```python
from build123d import *

# Parameters (mm, degrees)
BOSS_EXTRUDE1_DEPTH  = 3
SKETCH2_R            = 6
CUT_EXTRUDE1_DEPTH   = 4
M5_CLEARANCE_HOLE1_D = 5.5


with BuildPart() as part:
    # Sketch1 → Boss-Extrude1 (new body)
    with BuildSketch(Plane.XY):
        Polygon((-12.5, 55), (-32.5, 35), (-32.5, 2), (-30.5, 0), (30.5, 0), (32.5, 2), (32.5, 35), (12.5, 55), align=None)
    extrude(amount=BOSS_EXTRUDE1_DEPTH)

    # Sketch2 → Cut-Extrude1 (cut, through all)
    with BuildSketch(Plane.XY):
        with Locations((0, 40)):
            Circle(SKETCH2_R)
    extrude(amount=CUT_EXTRUDE1_DEPTH, mode=Mode.SUBTRACT)

    # M5 Clearance Hole1 (through all)
    with Locations(Plane.XY.offset(3)):
        with Locations((-22.5, 14.5), (22.5, 14.5)):
            Hole(M5_CLEARANCE_HOLE1_D / 2)


solid = part.part
```
Can you work these out from the model? Positions are in its coordinate system, mm. Give positions to 0.01 mm unless a question says otherwise; leave off trailing zeros. Write each loop counter-clockwise with the first axis right and the second up, starting at its lowest first coordinate (ties: lowest second). Pieces come first, ordered by that corner, then holes. Notation, with made-up numbers: (84.5, -13.5) -> (88.5, -13.5) arc R14 cw to (88.5, -4.5) -> close; hole circle Ø1 at (32, 80). An arc over 180 degrees is marked (long way). Write item = value, one per line.
(1) Suppose I cut it at B-B on x = -22.5. Write out the boundary of the cut face in (y, z).
Worked out:
outline = (0, 0) -> (11.75, 0) -> (11.75, 3) -> (0, 3) -> close; (17.25, 0) -> (45, 0) -> (45, 3) -> (17.25, 3) -> close
(2) I'm going to push a flat-ended pin straight in: P1, Ø1.5, axis at x = -20.5, z = 1.5, coming from the +Y side. Where does the tip first touch, or does it pass through?
Worked out:
P1 = 47.75
(3) Suppose I cut it at C-C on z = 1.15. Write out the boundary of the cut face in (x, y), then the cut area to 3 significant figures.
Worked out:
outline = (-32.5, 2) -> (-30.5, 0) -> (30.5, 0) -> (32.5, 2) -> (32.5, 35) -> (12.5, 55) -> (-12.5, 55) -> (-32.5, 35) -> close; hole circle Ø5.5 at (-22.5, 14.5); hole circle Ø12 at (0, 40); hole circle Ø5.5 at (22.5, 14.5)
area = 3,010 mm^2
(4) Suppose I cut it at A-A on y = 40. Write out the boundary of the cut face in (x, z), then the cut area to 3 significant figures.
Worked out:
outline = (-27.5, 0) -> (-6, 0) -> (-6, 3) -> (-27.5, 3) -> close; (6, 0) -> (27.5, 0) -> (27.5, 3) -> (6, 3) -> close
area = 129 mm^2
(5) I need wall thicknesses on probe 1 along X at (y, z) = (12, 1.4); probe 2 along Y at (x, z) = (0, 2.05); probe 3 along Y at (x, z) = (21, 1.2). Which ranges of each line are inside material? Lowest first, please. Write a range as from..to.
Worked out:
probe_1 = -32.5..-23.65, -21.35..21.35, 23.65..32.5
probe_2 = 0..34, 46..55
probe_3 = 0..12.2, 16.8..46.5
(6) Suppose I cut it at D-D on y = 14.5. Write out the boundary of the cut face in (x, z).
Worked out:
outline = (-32.5, 0) -> (-25.25, 0) -> (-25.25, 3) -> (-32.5, 3) -> close; (-19.75, 0) -> (19.75, 0) -> (19.75, 3) -> (-19.75, 3) -> close; (25.25, 0) -> (32.5, 0) -> (32.5, 3) -> (25.25, 3) -> close
(7) Thinking about a two-plate mould opening in Y: for faces 1 (the face through (25.247, 14.621, 1.479)), 2 (the face through (0, 55, 1)), 3 (the face through (-19.753, 14.621, 1.479)), 4 (the face through (-32.5, 19, 1)), which applies, released by +Y, released by -Y, zero draft, split by the parting line, or undercut?
Worked out:
face_1 = undercut
face_2 = released by +Y
face_3 = undercut
face_4 = zero draft
